Job drawing, mm, ordinate dimensions from the low corner. One solid piece. Give positions to 0.01 mm unless a question says otherwise; leave off trailing zeros. Loops run counter-clockwise (first coordinate to the right, second up) from the corner with the lowest first, then second, coordinate; pieces in that order, holes last. Notation, with made-up numbers: (82, 19) -> (123, 19) arc R10 ccw to (123, 30) -> close; hole circle Ø5 at (-34.75, -38.75). An arc over 180 degrees is marked (long way). Answer as a JSON object with one key per item and string values. Group by question number.
Q1. Wall check: probe 1 along Z at (x, y) = (47, 0.7); probe 2 along Y at (x, z) = (27.5, 9). Give the ranges that are in metal, low to high. Write a range as from..to.
Q2. Band-saw the part on B-B, the plane x = 12. Write the cut outline in (y, z).
Q3. Band-saw the part on A-A, the plane x = 47. Write the cut outline in (y, z), plus the area to 3 significant figures.
Q4. Band-saw the part on D-D, the plane y = 2.75. Write the cut outline in (x, z).
Q5. Drop flat-ended pins along their axis: pin 1 (3 mm diameter, centred on x = 47, z = 3, fed in from +Y); pin 2 (0.9 mm diameter, centred on y = 3.5, z = 1.5, fed in from +X); pin 3 (5 mm diameter, centred on x = 3, z = 87, fed in from +Y). Give the stop position or say it passes through.
Q6. Band-saw the part on C-C, the plane z = 43.5. Write the cut outline in (x, y).
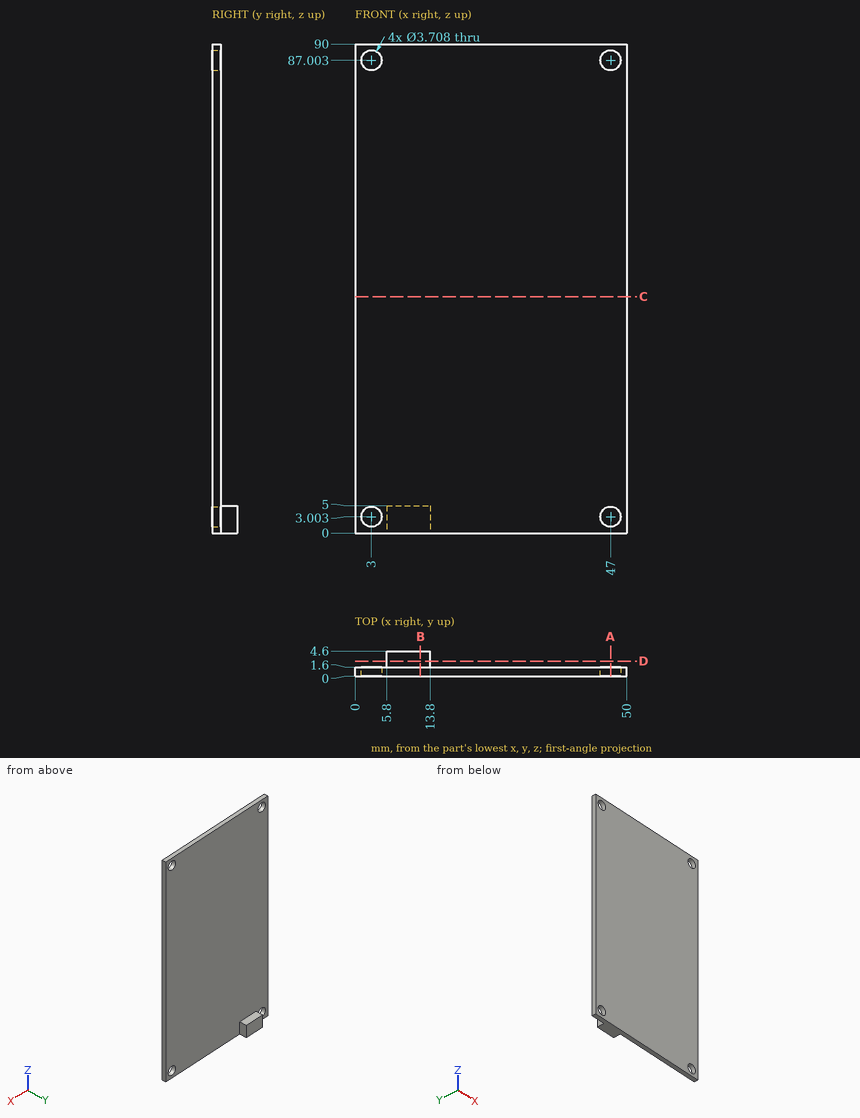
Worked answers:
{
 "1": {"probe 1": "0..1.15, 4.86..85.15, 88.86..90", "probe 2": "0..1.6"},
 "2": {"outline": "(0, 0) -> (4.6, 0) -> (4.6, 5) -> (1.6, 5) -> (1.6, 90) -> (0, 90) -> close"},
 "3": {"outline": "(0, 0) -> (1.6, 0) -> (1.6, 1.15) -> (0, 1.15) -> close; (0, 4.86) -> (1.6, 4.86) -> (1.6, 85.15) -> (0, 85.15) -> close; (0, 88.86) -> (1.6, 88.86) -> (1.6, 90) -> (0, 90) -> close", "area": "132 mm2"},
 "4": {"outline": "(5.8, 0) -> (13.8, 0) -> (13.8, 5) -> (5.8, 5) -> close"},
 "5": {"pin 1": "through", "pin 2": "x = 13.8", "pin 3": "y = 1.6"},
 "6": {"outline": "(0, 0) -> (50, 0) -> (50, 1.6) -> (0, 1.6) -> close"}
}
